from build123d import *

# Parameters (mm, degrees)
F3_DEPTH = 75
F4_T     = -3
F5_R     = 5


with BuildPart() as f3:
    # F2 (on Right) → F3 (new body, symmetric)
    with BuildSketch(Plane.YZ):
        Polygon((0, 75), (0, 0), (0, -75), (40, -75), (40, -35), (20, -15), (20, 75), align=None)
    extrude(amount=F3_DEPTH, both=True)

    # F4
    f4_openings = [f3.faces().sort_by_distance(p)[0] for p in [
        (0, 20, -75),
    ]]
    offset(amount=F4_T, openings=f4_openings, kind=Kind.INTERSECTION)

    # F5
    f5_edges = [f3.edges().sort_by_distance(p)[0] for p in [
        (72, 3, -1.5),
        (-72, 3, -1.5),
        (-75, 10, 75),
        (-75, 20, 30),
        (-75, 30, -25),
        (-75, 40, -55),
        (0, 20, 75),
        (0, 0, 75),
        (75, 10, 75),
        (75, 20, 30),
        (75, 30, -25),
        (75, 40, -55),
        (0, 40, -35),
        (0, 20, -15),
    ]]
    fillet(f5_edges, radius=F5_R)


solid = f3.part
Verification items for the finished model (mm, model axes). A direction names the side the tool comes from. Give positions to 0.01 mm unless a question says otherwise; leave off trailing zeros. Loops run counter-clockwise (first coordinate to the right, second up) from the corner with the lowest first, then second, coordinate; pieces in that order, holes last.
1) Sectioned sample at A-A, the plane z = -42.5. Enter the section's corners in (x, y).
2) Sectioned sample at C-C, the plane x = 41.5. Enter the section's corners in (y, z).
3) Draft check along Y on faces 1 (the flat face through (1, 10, 72)), 2 (the cylindrical face through (-1, 18, 74)), 3 (the cylindrical face through (73, 7, 74)). Enter one of: pulls with the +Y half, pulls with the -Y half, needs draft (parallel to the pull), parting line crosses it, or undercut.
4) Sectioned sample at D-D, the plane z = -6.5. Enter the section's corners in (x, y), then the cut area to 3 significant figures.
5) Depth check by flat-ended pin: pin 1 Ø2 at (x, y) = (-35.5, 31.5) entering from -Z; pin 2 Ø14.5 at (y, z) = (24.5, 6) entering from +X; pin 3 Ø4 at (x, z) = (-4, 58.5) entering from +Y. Enter the tip coordinate at first touch or a pass-through.
6) Set-up check for faces 4 (the cylindrical face through (-0.98, 20.37, -14.82)), 5 (the cylindrical face through (73, 19, 29)), 6 (the flat face through (-72, 16, -17)): record each of +Z, -Z, +X, -X, +Y, -Y from which the full face is reachable in a straight line by a thin tool's end or side.
7) Sectioned sample at B-B, the plane y = 10.5. Enter the section's corners in (x, z), then the cut area to 3 significant figures.
8) Thickness scan on line 1 along Y through (x, z) = (4, -1); line 2 along Y through (x, z) = (-37.5, -52.5); line 3 along X through (y, z) = (14, 48). Record the ranges inside material, lowest first.
Answers:
1. outline: (-75, 0) - (75, 0) - (75, 35) arc R5 ccw to (70, 40) - (-70, 40) arc R5 ccw to (-75, 35) - close; hole (-72, 8) arc R5 ccw to (-67, 3) - (67, 3) arc R5 ccw to (72, 8) - (72, 37) - (-72, 37) - close
2. outline: (0, -75) - (3, -75) - (3, 72) - (17, 72) - (17, -16.24) - (37, -36.24) - (37, -75) - (40, -75) - (40, -37.07) arc R5 ccw to (38.54, -33.54) - (21.46, -16.46) arc R5 cw to (20, -12.93) - (20, 70) arc R5 ccw to (15, 75) - (5, 75) arc R5 ccw to (0, 70) - close
3. face 1: undercut
3. face 2: pulls with the +Y half
3. face 3: needs draft
4. outline: (-75, 0) - (75, 0) - (75, 15) arc R5 ccw to (70, 20) - (-70, 20) arc R5 ccw to (-75, 15) - close; hole (-72, 8) arc R5 ccw to (-67, 3) - (67, 3) arc R5 ccw to (72, 8) - (72, 17) - (-72, 17) - close
4. area: 984 mm2
5. pin 1: stops at z = -31.74
5. pin 2: stops at x = 74.47
5. pin 3: stops at y = 20
6. face 4: +Z, +X, -X, +Y
6. face 5: +Z, +X, +Y
6. face 6: -Z
7. outline: (-75, -75) - (-72, -75) - (-72, 72) - (72, 72) - (72, -75) - (75, -75) - (75, 70) arc R5 ccw to (70, 75) - (-70, 75) arc R5 ccw to (-75, 70) - close
7. area: 1,320 mm2
8. line 1: y = 0 to 3, 17 to 20
8. line 2: y = 0 to 3, 37 to 40
8. line 3: x = -75 to -72, 72 to 75
